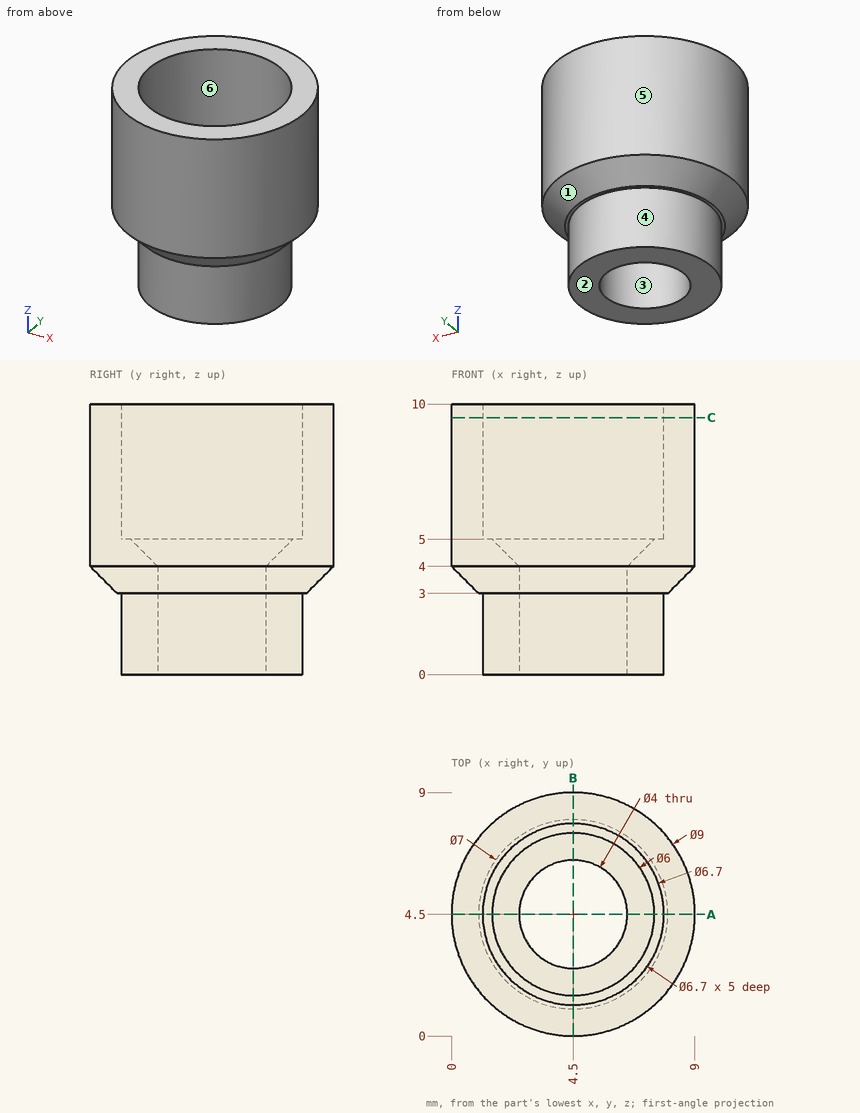
Here's the drawing with two shaded views (mm, measured from the low corner). I have some questions. A direction names the side the tool comes from. Round coordinates to 2 decimals unless told otherwise and drop trailing zeros. Order: outer loops, then holes, each group sorted by start corner. A loop starts at its lowest first (then second) coordinate and runs counter-clockwise, first axis right, second up. Notation, with made-up numbers: M 6,68.5 L 20,68.5 A23 cw 20,100.5 Z; hole C 89.25,-26 d4. An arc over 180 degrees is marked long. Use CSV: the item, a comma, the result in double quotes.
1) I need wall thicknesses on line 1 along Y through (x, z) = (4.5, 1.4); line 2 along Y through (x, z) = (4.5, 6.1); line 3 along Z through (x, y) = (7.75, 4.5). Which ranges of each line are inside material? Lowest first, please. Write a range as [from, to].
Taken from the geometry:
line 1,"[1.15, 2.5], [6.5, 7.85]"
line 2,"[0, 1.15], [7.85, 9]"
line 3,"[0, 5]"
2) On a 3-axis mill with a long thin cutter (end or side, diameter ignored), from which of +Z, -Z, +X, -X, +Y, -Y can I reach the whole of each face in a straight line? I mean the marked faces 4, 5 and 6. Say none if no direction works.
Taken from the geometry:
face 4,"-Z"
face 5,"+Z, -Z"
face 6,"+Z"
3) If we mould it in two halves opening along X, with no side actions, what happens to the marked faces 1, 2 and 3? For each: pulls with the +X half, pulls with the -X half, needs draft (parallel to the pull), parting line crosses it, or undercut.
Taken from the geometry:
face 1,"parting line crosses it"
face 2,"needs draft"
face 3,"undercut"
4) I'm going to push flat-ended pins straight in: P1, Ø1.5, axis at y = 7, z = 3, coming from the +X side; P2, Ø2, axis at y = 5, z = 7, coming from the -X side; P3, Ø1, axis at y = 7, z = 1.5, coming from the -X side; P4, Ø1.5, axis at x = 1, z = 3.5, coming from the -Y side. Where does each tip first touch, or does it pass through?
Taken from the geometry:
P1,"x = 8.07"
P2,"x = 0"
P3,"x = 1.81"
P4,"y = 1.09"
5) I want a section at A-A (y = 4.5). List the corners of the cut face in (x, z) for me.
Taken from the geometry:
outline,"M 0,4 L 1,3 L 1.15,3 L 1.15,0 L 2.5,0 L 2.5,4 L 1.5,5 L 1.15,5 L 1.15,10 L 0,10 Z; M 6.5,0 L 7.85,0 L 7.85,3 L 8,3 L 9,4 L 9,10 L 7.85,10 L 7.85,5 L 7.5,5 L 6.5,4 Z"
6) I want a section at C-C (z = 9.5). List the corners of the cut face in (x, y) for me, then the cut area to 3 significant figures.
Taken from the geometry:
outline,"C 4.5,4.5 d9; hole C 4.5,4.5 d6.7"
area,"28.4 mm^2"
